Answer from the drawing. Dimensions are ordinates in mm from the lowest x, y and z of the part. A direction names the side the tool comes from. Round coordinates to 2 decimals unless told otherwise and drop trailing zeros. Write each loop counter-clockwise with the first axis right and the second up, starting at its lowest first coordinate (ties: lowest second). Pieces come first, ordered by that corner, then holes. Notation, with made-up numbers: M 58.25,2.5 L 109.25,2.5 A29 cw 109.25,34.5 Z; hole C -38.75,80 d10. An arc over 180 degrees is marked long. Answer as CSV lines item,"result". Start each with the question number.
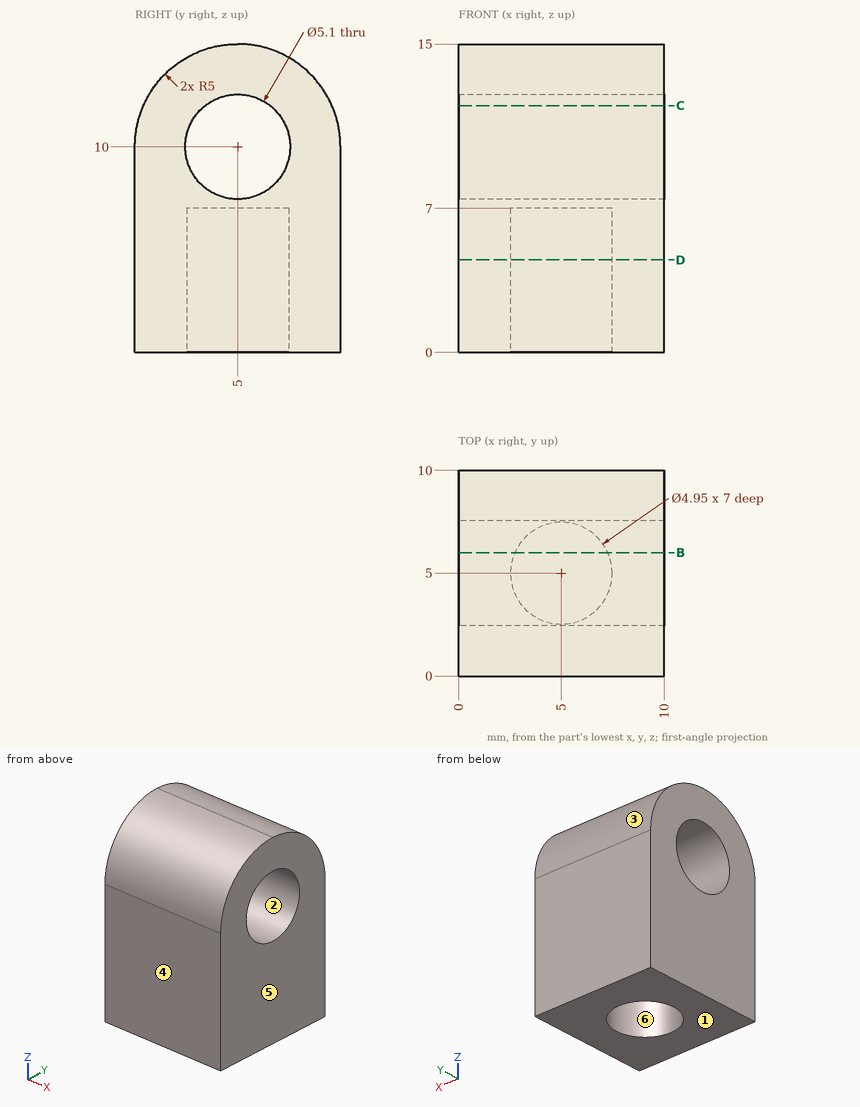
Q1. Find section D-D (z = 4.5). Determine the outline of the cut face in (x, y) (3 decimals).
Q2. For the marked faces 5 and 6, determine the directions among +Z, -Z, +X, -X, +Y, -Y from which every point of the face is accessible in a straight line to the end or side of a thin tool.
Q3. Each of these flat-tipped pins is pushed along its axis until it touches: P1, Ø1.5, axis at x = 4.5, y = 6, coming from the +Z side; P2, Ø4, axis at y = 5, z = 10, coming from the -X side. Where does it stop, or does it pass through?
Q4. Find section C-C (z = 12). Determine the outline of the cut face in (x, y), plus the area to 3 significant figures.
Q5. Find section B-B (y = 6). Determine the outline of the cut face in (x, z), plus the area to 3 significant figures.
Q6. The mould has two halves that part along Z. Classify the marked faces 1, 2, 3 and 4: +Z half, -Z half, draft (parallel to the pull), parting line (faces both ways), or undercut.
Q7. Straight lines are drawn through the part: L1, parallel to Y at x = 5.25, z = 10; L2, parallel to Z at x = 5, y = 5.5 (1 decimal); L3, parallel to X at y = 5.75, z = 1.5. For each, find the intervals that lie inside material, in ascending order.
Reported:
1,outline,"M 0,0 L 10,0 L 10,10 L 0,10 Z; hole C 5,5 d4.95"
2,face 5,"+Z, -Z, +X, +Y, -Y"
2,face 6,"-Z"
3,P1,"stops at z = 14.99"
3,P2,"passes through"
4,outline,"M 0,0.42 L 10,0.42 L 10,3.42 L 0,3.42 Z; M 0,6.58 L 10,6.58 L 10,9.58 L 0,9.58 Z"
4,area,"60.0 mm2"
5,outline,"M 0,0 L 2.74,0 L 2.74,7 L 7.26,7 L 7.26,0 L 10,0 L 10,7.65 L 0,7.65 Z; M 0,12.35 L 10,12.35 L 10,14.9 L 0,14.9 Z"
5,area,"70.4 mm2"
6,face 1,"-Z half"
6,face 2,"undercut"
6,face 3,"+Z half"
6,face 4,"draft"
7,L1,"y = 0 to 2.45, 7.55 to 10"
7,L2,"z = 7 to 7.5, 12.5 to 15"
7,L3,"x = 0 to 2.64, 7.36 to 10"
